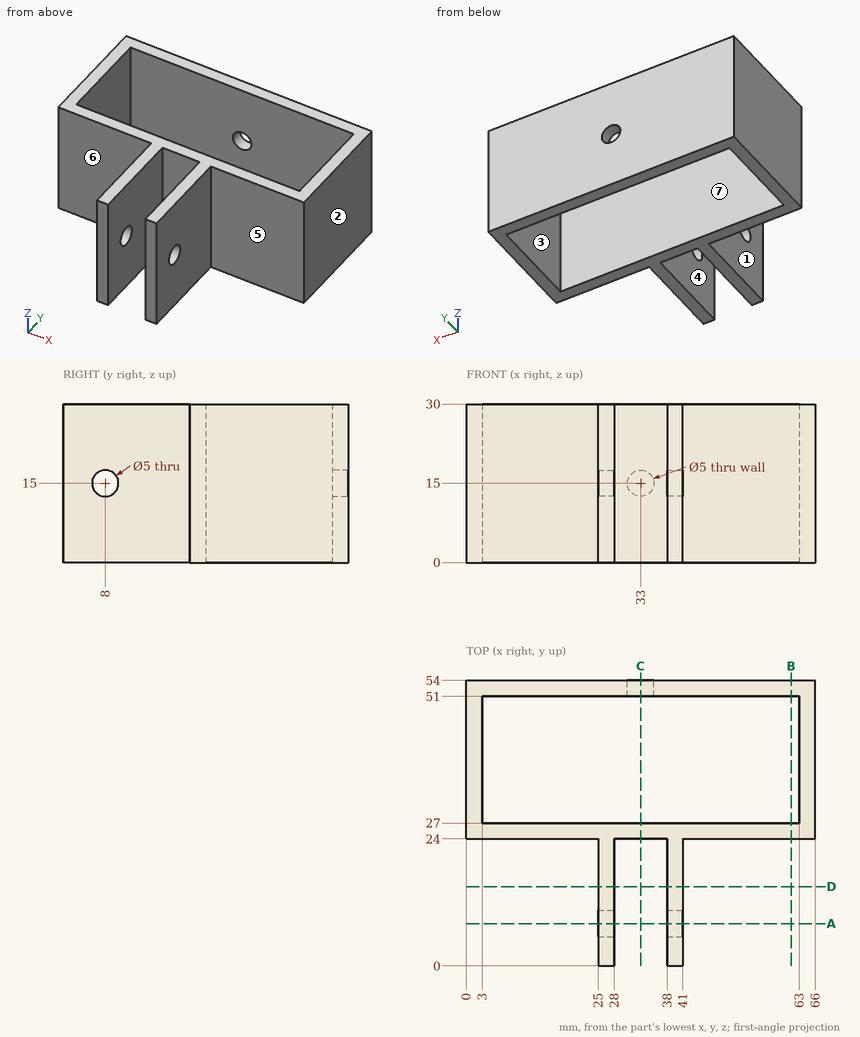
For this review, use the dimensioned drawing (mm, ordinates from the lowest corner) and the shaded views. A direction names the side the tool comes from. Round coordinates to 2 decimals unless told otherwise and drop trailing zeros. Write each loop counter-clockwise with the first axis right and the second up, starting at its lowest first coordinate (ties: lowest second). Pieces come first, ordered by that corner, then holes. Notation, with made-up numbers: (68.5, 82.5) - (84.5, 82.5) arc R16 cw to (84.5, 93.5) - close; hole circle Ø11 at (83.25, 26.25). An arc over 180 degrees is marked (long way). Answer as a JSON object with one key per item and string values.
1. We need section B-B on x = 61.5. Give the boundary of the cut face in (y, z), then the cut area to 3 significant figures.
Response values:
{"outline": "(24, 0) - (27, 0) - (27, 30) - (24, 30) - close; (51, 0) - (54, 0) - (54, 30) - (51, 30) - close", "area": "180 mm2"}
2. We need section D-D on y = 15. Give the boundary of the cut face in (x, z).
Response values:
{"outline": "(25, 0) - (28, 0) - (28, 30) - (25, 30) - close; (38, 0) - (41, 0) - (41, 30) - (38, 30) - close"}
3. We need section C-C on x = 33. Give the boundary of the cut face in (y, z), then the cut area to 3 significant figures.
Response values:
{"outline": "(24, 0) - (27, 0) - (27, 30) - (24, 30) - close; (51, 0) - (54, 0) - (54, 12.5) - (51, 12.5) - close; (51, 17.5) - (54, 17.5) - (54, 30) - (51, 30) - close", "area": "165 mm2"}
4. Tool access review of the marked faces 4, 5, 6 and 7: name each direction out of +Z, -Z, +X, -X, +Y, -Y from which nothing blocks a thin tool from reaching the whole face with its end or side.
Response values:
{"face 4": "+Z, -Z, -Y", "face 5": "+Z, -Z, +X, -Y", "face 6": "+Z, -Z, -X, -Y", "face 7": "+Z, -Z"}
5. For pin 1 Ø12 at (y, z) = (15.5, 15) entering from -X; pin 2 Ø7 at (y, z) = (6, 18.5) entering from +X; pin 3 Ø12.5 at (x, z) = (8.5, 20) entering from -Y, all flat-tipped, find the tip position at first contact; note any pin that passes through.
Response values:
{"pin 1": "stops at x = 25", "pin 2": "stops at x = 41", "pin 3": "stops at y = 24"}
6. Draft analysis for pull direction X (two halves, no side actions). For the marked faces 1, 2 and 3, state which applies: +X half, -X half, draft (parallel to the pull), parting line (faces both ways), or undercut.
Response values:
{"face 1": "-X half", "face 2": "+X half", "face 3": "undercut"}
7. To check wall thickness, follow line 1 along Y through (x, z) = (38.65, 15); line 2 along Y through (x, z) = (59, 24.5); line 3 along X through (y, z) = (38.5, 8). State the ranges of each line that lie inside material, in increasing order.
Response values:
{"line 1": "y = 0 to 5.5, 10.5 to 27, 51 to 54", "line 2": "y = 24 to 27, 51 to 54", "line 3": "x = 0 to 3, 63 to 66"}
8. We need section A-A on y = 8. Give the boundary of the cut face in (x, z), then the cut area to 3 significant figures.
Response values:
{"outline": "(25, 0) - (28, 0) - (28, 12.5) - (25, 12.5) - close; (25, 17.5) - (28, 17.5) - (28, 30) - (25, 30) - close; (38, 0) - (41, 0) - (41, 12.5) - (38, 12.5) - close; (38, 17.5) - (41, 17.5) - (41, 30) - (38, 30) - close", "area": "150 mm2"}
